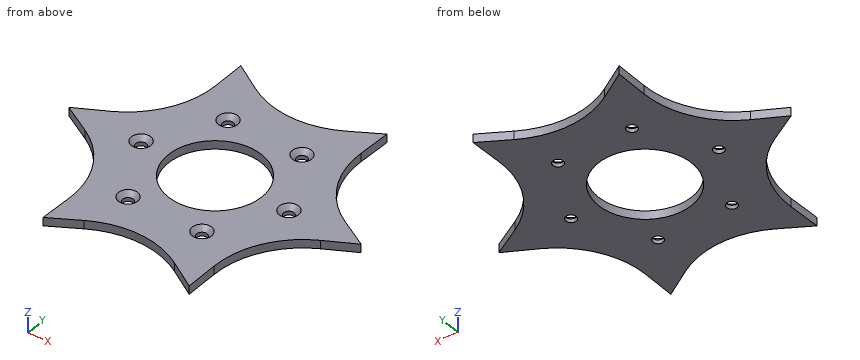
from build123d import *

# Parameters (mm, degrees)
SKETCH7_R           = 25
BOSS_EXTRUDE5_DEPTH = 4.5
CIRPATTERN1_COUNT   = 6


with BuildPart() as part:
    # Sketch7 → Boss-Extrude5 (new body)
    with BuildSketch(Plane.XY.offset(62.545612614)):
        with BuildLine():
            Line((-39.557386288, -68.515402865), (-24.43179769, -59.410864919))
            ThreePointArc((-24.43179769, -59.410864919), (0, -52.625), (24.43179769, -59.410864919))
            Line((24.43179769, -59.410864919), (39.557386288, -68.515402865))
            Line((39.557386288, -68.515402865), (39.235419436, -50.863989919))
            ThreePointArc((39.235419436, -50.863989919), (45.574586874, -26.3125), (63.667217125, -8.546875))
            Line((63.667217125, -8.546875), (79.114772576, 0))
            Line((79.114772576, 0), (63.667217125, 8.546875))
            ThreePointArc((63.667217125, 8.546875), (45.574586874, 26.3125), (39.235419436, 50.863989919))
            Line((39.235419436, 50.863989919), (39.557386288, 68.515402865))
            Line((39.557386288, 68.515402865), (24.43179769, 59.410864919))
            ThreePointArc((24.43179769, 59.410864919), (0, 52.625), (-24.43179769, 59.410864919))
            Line((-24.43179769, 59.410864919), (-39.557386288, 68.515402865))
            Line((-39.557386288, 68.515402865), (-39.235419436, 50.863989919))
            ThreePointArc((-39.235419436, 50.863989919), (-45.574586874, 26.3125), (-63.667217125, 8.546875))
            Line((-63.667217125, 8.546875), (-79.114772576, 0))
            Line((-79.114772576, 0), (-63.667217125, -8.546875))
            ThreePointArc((-63.667217125, -8.546875), (-45.574586874, -26.3125), (-39.235419436, -50.863989919))
            Line((-39.235419436, -50.863989919), (-39.557386288, -68.515402865))
        make_face()
        Circle(SKETCH7_R, mode=Mode.SUBTRACT)
    extrude(amount=BOSS_EXTRUDE5_DEPTH)

    # Sketch11 → CSK for M5 Flat Head Machine Screw1 (revolve, cut)
    with BuildSketch(Plane(origin=(-40, 0, 67.045612614), x_dir=(0, -1, 0), z_dir=(1, 0, 0))):
        Polygon((0, 0), (0, 4.5), (2.75, 4.5), (2.75, 2.45), (5.2, 0), align=None)
    csk_for_m5_flat_head_machine_screw1 = revolve(axis=Axis((-40, 0, 73.395612614), (0, 0, -1)), mode=Mode.SUBTRACT)

    # CirPattern1: CSK for M5 Flat Head Machine Screw1 ×6 about axis
    cirpattern1_axis = Axis((0, 0, 0), (0, 0, 1))
    for i in range(1, CIRPATTERN1_COUNT):
        add(csk_for_m5_flat_head_machine_screw1.rotate(cirpattern1_axis, i * 360 / CIRPATTERN1_COUNT), mode=Mode.SUBTRACT)


solid = part.part
Geometry check sheet. Reference: the model listing, model coordinates, mm. Give positions to 0.01 mm unless a question says otherwise; leave off trailing zeros. Order: outer loops, then holes, each group sorted by start corner. A loop starts at its lowest first (then second) coordinate and runs counter-clockwise, first axis right, second up. Notation, with made-up numbers: (-15, 63.25) - (39, 63.25) arc R31 ccw to (39, 90.25) - close; hole circle Ø9 at (27.25, -28.75). An arc over 180 degrees is marked (long way). Answer as a JSON object with one key per item and string values.
(1) Cross-section at B-B (z = 63.9). Record the cut outline in (x, y) (3 decimals), then the cut area to 3 significant figures.
Report:
{"outline": "(-79.115, 0) - (-63.667, -8.547) arc R47.375 cw to (-39.235, -50.864) - (-39.557, -68.515) - (-24.432, -59.411) arc R47.375 cw to (24.432, -59.411) - (39.557, -68.515) - (39.235, -50.864) arc R47.375 cw to (63.667, -8.547) - (79.115, 0) - (63.667, 8.547) arc R47.375 cw to (39.235, 50.864) - (39.557, 68.515) - (24.432, 59.411) arc R47.375 cw to (-24.432, 59.411) - (-39.557, 68.515) - (-39.235, 50.864) arc R47.375 cw to (-63.667, 8.547) - close; hole circle Ø5.5 at (-40, 0); hole circle Ø50 at (0, 0); hole circle Ø5.5 at (-20, -34.641); hole circle Ø5.5 at (-20, 34.641); hole circle Ø5.5 at (20, -34.641); hole circle Ø5.5 at (20, 34.641); hole circle Ø5.5 at (40, 0)", "area": "9,310 mm^2"}
(2) Cross-section at A-A (x = 20). Record the cut outline in (y, z).
Report:
{"outline": "(-57.05, 62.55) - (-37.39, 62.55) - (-37.39, 64.6) - (-39.84, 67.05) - (-57.05, 67.05) - close; (-31.89, 62.55) - (-15, 62.55) - (-15, 67.05) - (-29.44, 67.05) - (-31.89, 64.6) - close; (15, 62.55) - (31.89, 62.55) - (31.89, 64.6) - (29.44, 67.05) - (15, 67.05) - close; (37.39, 62.55) - (57.05, 62.55) - (57.05, 67.05) - (39.84, 67.05) - (37.39, 64.6) - close"}
(3) Cross-section at D-D (y = 27.5). Record the cut outline in (x, z), then the cut area to 3 significant figures.
Report:
{"outline": "(-44.91, 62.55) - (44.91, 62.55) - (44.91, 67.05) - (-44.91, 67.05) - close", "area": "404 mm^2"}
(4) Depth check by flat-ended pin: pin 1 Ø5 at (x, y) = (-20, -34.64) entering from -Z; pin 2 Ø2 at (y, z) = (-12.5, 63.5) entering from -X; pin 3 Ø2 at (y, z) = (-35, 66.5) entering from +X; pin 4 Ø1 at (x, z) = (-8, 63.5) entering from +Y. Enter the tip coordinate at first touch or a pass-through.
Report:
{"pin 1": "through", "pin 2": "x = -59", "pin 3": "x = 42.01", "pin 4": "y = 53.39"}
(5) Cross-section at C-C (y = -57.5). Record the cut outline in (x, z), then the cut area to 3 significant figures.
Report:
{"outline": "(-39.36, 62.55) - (-20.93, 62.55) - (-20.93, 67.05) - (-39.36, 67.05) - close; (20.93, 62.55) - (39.36, 62.55) - (39.36, 67.05) - (20.93, 67.05) - close", "area": "166 mm^2"}
(6) Material ranges on line 1 (Y direction, x = 19.5, z = 66.75); line 2 (Y direction, x = 0, z = 64.5) (3 decimals); line 3 (X direction, y = -37, z = 62.9), recorded low to high.
Report:
{"line 1": "-56.82 to -39.52, -29.76 to -15.64, 15.64 to 29.76, 39.52 to 56.82", "line 2": "-52.625 to -25, 25 to 52.625", "line 3": "-41.05 to -21.41, -18.59 to 18.59, 21.41 to 41.05"}
